Geometry: final body of the model. Coordinates: model frame, mm. Face numbers are marked on the shaded views. A direction names the side the tool comes from. Give positions to 0.01 mm unless a question says otherwise; leave off trailing zeros. Loops run counter-clockwise (first coordinate to the right, second up) from the corner with the lowest first, then second, coordinate; pieces in that order, holes last.
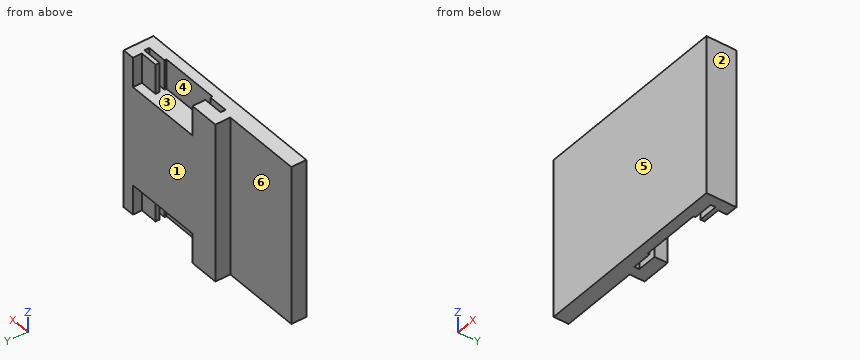
from build123d import *

# Parameters (mm, degrees)
SKETCH1_W               = 320
SKETCH1_H               = 160
BOSS_EXTRUDE1_DEPTH     = 20
SKETCH2_W               = 60
SKETCH2_H               = 30
CUT_EXTRUDE1_DEPTH      = 28
SKETCH3_W               = 20
SKETCH3_H               = 5
CUT_EXTRUDE3_DEPTH      = 30
MIRROR3_COPY_1_SKETCH_W = 60
MIRROR3_COPY_1_SKETCH_H = 30
MIRROR3_COPY_1_DEPTH    = 28
MIRROR3_COPY_2_SKETCH_W = 20
MIRROR3_COPY_2_SKETCH_H = 5
MIRROR3_COPY_2_DEPTH    = 30
SKETCH8_W               = 18
SKETCH8_H               = 9
CUT_EXTRUDE6_DEPTH      = 30
SKETCH9_W               = 18
SKETCH9_H               = 9
CUT_EXTRUDE7_DEPTH      = 30
SKETCH10_W              = 320
SKETCH10_H              = 160
BOSS_EXTRUDE2_DEPTH     = 10
CUT_EXTRUDE8_DEPTH      = 236


with BuildPart() as part:
    # Sketch1 → Boss-Extrude1 (new body)
    with BuildSketch(Plane(origin=(0, 0, 0), x_dir=(1, 0, 0), z_dir=(0, 1, 0))):
        Rectangle(SKETCH1_W, SKETCH1_H)
    extrude(amount=BOSS_EXTRUDE1_DEPTH)

    # Sketch2 → Cut-Extrude1 (cut)
    with BuildSketch(Plane(origin=(0, 20, 0), x_dir=(1, 0, 0), z_dir=(0, 1, 0))):
        with Locations((-100, -65)):
            Rectangle(SKETCH2_W, SKETCH2_H)
    cut_extrude1 = extrude(amount=-CUT_EXTRUDE1_DEPTH, mode=Mode.SUBTRACT)

    # Sketch3 → Cut-Extrude3 (cut)
    with BuildSketch(Plane.XY.offset(80)):
        with Locations((-140, 4.5)):
            Rectangle(SKETCH3_W, SKETCH3_H)
        with Locations((-60, 4.5)):
            Rectangle(SKETCH3_W, SKETCH3_H)
    cut_extrude3 = extrude(amount=-CUT_EXTRUDE3_DEPTH, mode=Mode.SUBTRACT)

    # Mirror2: Cut-Extrude1, Cut-Extrude3 across plane
    add(cut_extrude1.mirror(Plane(origin=(0, 0, 0), x_dir=(0, 0, 1), z_dir=(1, 0, 0))), mode=Mode.SUBTRACT)
    add(cut_extrude3.mirror(Plane(origin=(0, 0, 0), x_dir=(0, 0, 1), z_dir=(1, 0, 0))), mode=Mode.SUBTRACT)

    # Mirror3: Cut-Extrude1, Cut-Extrude3 across plane
    add(cut_extrude1.mirror(Plane.XY), mode=Mode.SUBTRACT)
    add(cut_extrude3.mirror(Plane.XY), mode=Mode.SUBTRACT)

    # Mirror3 copy 1 sketch → Mirror3 copy 1 (cut)
    with BuildSketch(Plane(origin=(0, 20, 0), x_dir=(-1, 0, 0), z_dir=(0, 1, 0))):
        with Locations((-100, -65)):
            Rectangle(MIRROR3_COPY_1_SKETCH_W, MIRROR3_COPY_1_SKETCH_H)
    extrude(amount=-MIRROR3_COPY_1_DEPTH, mode=Mode.SUBTRACT)

    # Mirror3 copy 2 sketch → Mirror3 copy 2 (cut)
    with BuildSketch(Plane(origin=(0, 0, -80), x_dir=(-1, 0, 0), z_dir=(0, 0, -1))):
        with Locations((-140, 4.5)):
            Rectangle(MIRROR3_COPY_2_SKETCH_W, MIRROR3_COPY_2_SKETCH_H)
        with Locations((-60, 4.5)):
            Rectangle(MIRROR3_COPY_2_SKETCH_W, MIRROR3_COPY_2_SKETCH_H)
    extrude(amount=-MIRROR3_COPY_2_DEPTH, mode=Mode.SUBTRACT)

    # Sketch8 → Cut-Extrude6 (cut)
    with BuildSketch(Plane(origin=(0, 0, -80), x_dir=(-1, 0, 0), z_dir=(0, 0, -1))):
        with Locations((-139, 15.5)):
            Rectangle(SKETCH8_W, SKETCH8_H)
    cut_extrude6 = extrude(amount=-CUT_EXTRUDE6_DEPTH, mode=Mode.SUBTRACT)

    # Sketch9 → Cut-Extrude7 (cut)
    with BuildSketch(Plane(origin=(0, 0, -80), x_dir=(-1, 0, 0), z_dir=(0, 0, -1))):
        with Locations((61, 15.5)):
            Rectangle(SKETCH9_W, SKETCH9_H)
    cut_extrude7 = extrude(amount=-CUT_EXTRUDE7_DEPTH, mode=Mode.SUBTRACT)

    # Sketch10 → Boss-Extrude2 (add)
    with BuildSketch(Plane.XZ):
        Rectangle(SKETCH10_W, SKETCH10_H)
    extrude(amount=BOSS_EXTRUDE2_DEPTH)

    # Mirror4: Cut-Extrude6, Cut-Extrude7 across plane
    add(cut_extrude6.mirror(Plane.XY), mode=Mode.SUBTRACT)
    add(cut_extrude7.mirror(Plane.XY), mode=Mode.SUBTRACT)

    # Sketch12 → Cut-Extrude8 (cut)
    with BuildSketch(Plane(origin=(0, 0, -80), x_dir=(-1, 0, 0), z_dir=(0, 0, -1))):
        Polygon((-40, 20), (-40, 5), (40, 5), (40, -10), (160, -10), (160, 20), align=None)
    extrude(amount=-CUT_EXTRUDE8_DEPTH, mode=Mode.SUBTRACT)


solid = part.part
Item 1: Section query D-D on x = 53. Return loops of the section in (y, z), plus the area to 3 significant figures.
Values follow:
outline: (-10, -80) - (2, -80) - (2, -50) - (7, -50) - (7, -80) - (20, -80) - (20, 80) - (7, 80) - (7, 50) - (2, 50) - (2, 80) - (-10, 80) - close
area: 4,500 mm2
Item 2: Pin query (flat end, axial travel): pin 1 (10 mm diameter, centred on x = 140, z = -64.5, fed in from +Y); pin 2 (4.5 mm diameter, centred on y = 9, z = -65.5, fed in from -X); pin 3 (5.5 mm diameter, centred on y = 5.5, z = -62, fed in from -X); pin 4 (2 mm diameter, centred on x = 77.5, y = 15, fed in from +Z). Return the tip coordinate at first contact, or that it passes through.
Values follow:
pin 1: stops at y = 11
pin 2: stops at x = 40
pin 3: stops at x = -40
pin 4: stops at z = 50
Item 3: Section query C-C on y = 14.25. Return loops of the section in (x, z), plus the area to 3 significant figures.
Values follow:
outline: (40, -80) - (70, -80) - (70, -50) - (148, -50) - (148, -80) - (160, -80) - (160, 80) - (148, 80) - (148, 50) - (70, 50) - (70, 80) - (40, 80) - close
area: 14,500 mm2
Item 4: Section query B-B on x = 98.5. Return loops of the section in (y, z).
Values follow:
outline: (-10, -80) - (0, -80) - (0, -50) - (20, -50) - (20, 50) - (0, 50) - (0, 80) - (-10, 80) - close
Item 5: Section query A-A on z = 65. Return loops of the section in (x, y), plus the area to 3 significant figures.
Values follow:
outline: (-40, -10) - (160, -10) - (160, 20) - (148, 20) - (148, 11) - (130, 11) - (130, 7) - (150, 7) - (150, 2) - (130, 2) - (130, 0) - (70, 0) - (70, 2) - (50, 2) - (50, 7) - (70, 7) - (70, 20) - (40, 20) - (40, 5) - (-40, 5) - close
area: 3,240 mm2
Item 6: Set-up query: the marked faces 4, 5 and 6. Return all of +Z, -Z, +X, -X, +Y, -Y with unobstructed straight access to the full face (end or side cutting, diameter ignored); none if empty.
Values follow:
face 4: +Z, +Y
face 5: +Z, -Z, +X, -X, -Y
face 6: +Z, -Z, -X, +Y
Item 7: Draft query along Y for the marked faces 1, 2 and 3. Return one class per face: +Y half, -Y half, draft (parallel to the pull), parting line (faces both ways), or undercut.
Values follow:
face 1: +Y half
face 2: draft
face 3: undercut
Item 8: Ray query, probe 1 along X at (y, z) = (18.5, 63); probe 2 along Y at (x, z) = (132, 69); probe 3 along X at (y, z) = (7.5, 55). Return the intervals inside material, ascending.
Values follow:
probe 1: x = 40 to 70, 148 to 160
probe 2: y = -10 to 2, 7 to 11
probe 3: x = 40 to 70, 130 to 160
